```python
from build123d import *

# Parameters (mm, degrees)
F0_W     = 60.325
F0_H     = 60.325
F1_DEPTH = 101.6
F3_W     = 15.875
F3_H     = 69.85
F4_DEPTH = 30.48
F5_W     = 15.875
F5_H     = 69.85
F6_DEPTH = 30.48
F7_R     = 6.35


with BuildPart() as f1:
    # F0 (on Top) → F1 (new body)
    with BuildSketch(Plane.XY):
        Rectangle(F0_W, F0_H)
    extrude(amount=F1_DEPTH)

    # F3 (on face) → F4 (cut)
    with BuildSketch(Plane.XZ.offset(30.1625)):
        with Locations((-9.525, 50.8)):
            Rectangle(F3_W, F3_H)
    extrude(amount=-F4_DEPTH, mode=Mode.SUBTRACT)

    # F5 (on face) → F6 (cut)
    with BuildSketch(Plane.YZ.offset(30.1625)):
        with Locations((9.525, 50.8)):
            Rectangle(F5_W, F5_H)
    extrude(amount=-F6_DEPTH, mode=Mode.SUBTRACT)

    # F7
    f7_edges = [f1.edges().sort_by_distance(p)[0] for p in [
        (-17.4625, -14.9225, 85.725),
        (-1.5875, -14.9225, 85.725),
        (-17.4625, -14.9225, 15.875),
        (-1.5875, -14.9225, 15.875),
        (14.9225, 17.4625, 85.725),
        (14.9225, 1.5875, 85.725),
        (14.9225, 1.5875, 15.875),
        (14.9225, 17.4625, 15.875),
    ]]
    fillet(f7_edges, radius=F7_R)


solid = f1.part
```
Part model, mm, in its own coordinate system. A direction names the side the tool comes from. Round coordinates to 2 decimals unless told otherwise and drop trailing zeros. Write each loop counter-clockwise with the first axis right and the second up, starting at its lowest first coordinate (ties: lowest second). Pieces come first, ordered by that corner, then holes. Notation, with made-up numbers: M -37,-10.5 L 15,-10.5 A16 ccw 15,0.5 Z; hole C 6.5,-11.5 d5. An arc over 180 degrees is marked long. Answer as CSV lines item,"result". Start each with the question number.
1) Band-saw the part on C-C (z = 38). List the corners of the cut face in (x, y), then the cut area to 3 significant figures.
2) Which spindle directions (+Z, -Z, +X, -X, +Y, -Y) get a long thin tool onto all of the face, cutting with end or side? Do faces 4 (the face through (-30.162, 0, 50)), 5 (the face through (15, 10, 85.725)), 6 (the face through (-3.4, -14.71, 17.78)). Say none if no direction does.
3) Drop a flat-ended pin along its axis: pin 1 (12.5 mm diameter, centred on y = 8.5, z = 40, fed in from +X). Give the stop position or say it passes through.
4) Band-saw the part on D-D (x = -3.5). List the corners of the cut face in (y, z), then the cut area to 3 significant figures.
5) Drill centre lines: L1, parallel to Z at x = 6, y = 9 (3 decimals); L2, parallel to X at y = -3.5, z = 46.5; L3, parallel to Y at x = 1, z = 79. Where is each one in solid material? Low to high.
6) Mould opens along X. For faces 1 (the face through (14.71, 3.4, 17.78)), 2 (the face through (30.162, 0, 50)), 3 (the face through (-15.65, -14.71, 83.82)) say: +X half, -X half, draft (parallel to the pull), parting line (faces both ways), or undercut.
Worked out:
1,outline,"M -30.16,-30.16 L -17.46,-30.16 L -17.46,0.32 L -1.59,0.32 L -1.59,-30.16 L 30.16,-30.16 L 30.16,1.59 L -0.32,1.59 L -0.32,17.46 L 30.16,17.46 L 30.16,30.16 L -30.16,30.16 Z"
1,area,"2,670 mm²"
2,face 4,"+Z, -Z, -X, +Y, -Y"
2,face 5,"+X"
2,face 6,"-Y"
3,pin 1,"x = -0.32"
4,outline,"M -30.16,0 L 30.16,0 L 30.16,101.6 L -30.16,101.6 L -30.16,83.92 L 0.32,83.92 L 0.32,17.68 L -30.16,17.68 Z"
4,area,"4,110 mm²"
5,L1,"0 to 15.875, 85.725 to 101.6"
5,L2,"-30.16 to -17.46, -1.59 to 30.16"
5,L3,"-30.16 to 1.59, 17.46 to 30.16"
6,face 1,"draft"
6,face 2,"+X half"
6,face 3,"undercut"
